Design review of the part built by this model. Coordinates are the model's own, in mm. A direction names the side the tool comes from. Round coordinates to 2 decimals unless told otherwise and drop trailing zeros. Order: outer loops, then holes, each group sorted by start corner. A loop starts at its lowest first (then second) coordinate and runs counter-clockwise, first axis right, second up. Notation, with made-up numbers: M -24.5,49.5 L 13.5,49.5 A14 cw 13.5,71.5 Z; hole C 62.5,-11.5 d3. An arc over 180 degrees is marked long. Write each question's results on one line, items separated by ' | '. Start each with the question number.
Item 1: Take a section at B-B, the plane x = 0. Write out the cut boundary in (y, z), plus the area to 3 significant figures.
Item 2: Take a section at A-A, the plane z = 8.5. Write out the cut boundary in (x, y), plus the area to 3 significant figures.
Item 3: Take a section at D-D, the plane x = 24.5. Write out the cut boundary in (y, z).
Item 4: Machinability: for faces 1 (the flat face through (20, 30, 5)), 2 (the flat face through (-20, 30, 5)), 3 (the flat face through (-30, -5, 5)), which of the approach directions +Z, -Z, +X, -X, +Y, -Y give a long, thin tool a straight path to every point of the face, cutting with its end or side? Answer none if there is none.
Item 5: The part is to be moulded in two halves that separate along Y. For faces 4 (the cylindrical face through (-2.17, 30.24, 4.93)), 5 (the flat face through (0, 6, 10)), 6 (the flat face through (0, -30, 5)), say which applies: +Y half, -Y half, draft (parallel to the pull), parting line (faces both ways), or undercut.
Item 6: Take a section at C-C, the plane y = 45. Write out the cut boundary in (x, z), plus the area to 3 significant figures.
Item 7: Wall thickness on line 1 (Y direction, x = 0, z = 7); line 2 (X direction, y = 42, z = 2.5); line 3 (Y direction, x = -24, z = 6.5): over which ranges is each line inside the solid? List them lowest first. Write a range as [from, to].
Item 8: Clearance check with flat-ended pins moving along their axes: pin 1 (3 mm diameter, centred on y = 34.5, z = 3.5, fed in from -X); pin 2 (5 mm diameter, centred on x = 26.5, z = 3, fed in from +Y). State where each tip first meets the part, or that it passes through.
```python
from build123d import *

# Parameters (mm, degrees)
BOSS_EXTRUDE1_DEPTH = 10
SKETCH2_R           = 10
BOSS_EXTRUDE2_DEPTH = 20
SKETCH3_W           = 60
SKETCH3_H           = 30
BOSS_EXTRUDE3_DEPTH = 10
CUT_EXTRUDE1_START  = -30
SKETCH4_R           = 10
CUT_EXTRUDE1_DEPTH  = 30


with BuildPart() as part:
    # Sketch1 → Boss-Extrude1 (new body)
    with BuildSketch(Plane.XY):
        with BuildLine():
            Line((-30, 0), (30, 0))
            Line((30, 0), (30, 20))
            Line((30, 20), (20, 20))
            Line((20, 20), (20, 40))
            ThreePointArc((20, 40), (0, 60), (-20, 40))
            Line((-20, 40), (-20, 20))
            Line((-20, 20), (-30, 20))
            Line((-30, 20), (-30, 0))
        make_face()
    extrude(amount=BOSS_EXTRUDE1_DEPTH)

    # Sketch2 → Boss-Extrude2 (add)
    with BuildSketch(Plane.XY.offset(10)):
        with Locations((0, 40)):
            Circle(SKETCH2_R)
    extrude(amount=BOSS_EXTRUDE2_DEPTH)

    # Sketch3 → Boss-Extrude3 (add)
    with BuildSketch(Plane.XY.offset(10)):
        with Locations((0, -15)):
            Rectangle(SKETCH3_W, SKETCH3_H)
    extrude(amount=-BOSS_EXTRUDE3_DEPTH)

    # Sketch4 → Cut-Extrude1 (cut)
    with BuildSketch(Plane.XY.offset(30).offset(CUT_EXTRUDE1_START)):
        with Locations((0, 40)):
            Circle(SKETCH4_R)
    extrude(amount=CUT_EXTRUDE1_DEPTH, mode=Mode.SUBTRACT)


solid = part.part
```
Results list:
1) outline: M -30,0 L 30,0 L 30,10 L -30,10 Z; M 50,0 L 60,0 L 60,10 L 50,10 Z | area: 700 mm²
2) outline: M -30,-30 L 30,-30 L 30,20 L 20,20 L 20,40 A20 ccw -20,40 L -20,20 L -30,20 Z; hole C 0,40 d20 | area: 4,110 mm²
3) outline: M -30,0 L 20,0 L 20,10 L -30,10 Z
4) face 1: +Z, -Z, +X, +Y | face 2: +Z, -Z, -X, +Y | face 3: +Z, -Z, -X, +Y, -Y
5) face 4: undercut | face 5: draft | face 6: -Y half
6) outline: M -19.36,0 L -8.66,0 L -8.66,10 L -19.36,10 Z; M 8.66,0 L 19.36,0 L 19.36,10 L 8.66,10 Z | area: 214 mm²
7) line 1: [-30, 30], [50, 60] | line 2: [-19.9, -9.8], [9.8, 19.9] | line 3: [-30, 20]
8) pin 1: x = -20 | pin 2: y = 20
